```python
from build123d import *

# Parameters (mm, degrees)
SKETCH1_W           = 40
SKETCH1_H           = 25
BOSS_EXTRUDE1_DEPTH = 2
CUT_EXTRUDE1_REACH  = 25.67
SKETCH2_R           = 1.55


with BuildPart() as part:
    # Sketch1 → Boss-Extrude1 (new body)
    with BuildSketch(Plane.XY):
        Rectangle(SKETCH1_W, SKETCH1_H)
    extrude(amount=BOSS_EXTRUDE1_DEPTH)

    # Sketch2 → Cut-Extrude1 (cut, up to next)
    with BuildSketch(Plane.XY.offset(2), mode=Mode.PRIVATE) as cut_extrude1_sk1:
        with Locations((-15, 7.5)):
            Circle(SKETCH2_R)
    cut_extrude1_tool1 = extrude(cut_extrude1_sk1.sketch, amount=-CUT_EXTRUDE1_REACH, mode=Mode.PRIVATE) & part.part
    # Sketch2 → Cut-Extrude1 (cut, up to next)
    with BuildSketch(Plane.XY.offset(2), mode=Mode.PRIVATE) as cut_extrude1_sk2:
        with Locations((-15, 0)):
            Circle(SKETCH2_R)
    cut_extrude1_tool2 = extrude(cut_extrude1_sk2.sketch, amount=-CUT_EXTRUDE1_REACH, mode=Mode.PRIVATE) & part.part
    # Sketch2 → Cut-Extrude1 (cut, up to next)
    with BuildSketch(Plane.XY.offset(2), mode=Mode.PRIVATE) as cut_extrude1_sk3:
        with Locations((-15, -7.5)):
            Circle(SKETCH2_R)
    cut_extrude1_tool3 = extrude(cut_extrude1_sk3.sketch, amount=-CUT_EXTRUDE1_REACH, mode=Mode.PRIVATE) & part.part
    # Sketch2 → Cut-Extrude1 (cut, up to next)
    with BuildSketch(Plane.XY.offset(2), mode=Mode.PRIVATE) as cut_extrude1_sk4:
        with Locations((15, -7.5)):
            Circle(SKETCH2_R)
    cut_extrude1_tool4 = extrude(cut_extrude1_sk4.sketch, amount=-CUT_EXTRUDE1_REACH, mode=Mode.PRIVATE) & part.part
    # Sketch2 → Cut-Extrude1 (cut, up to next)
    with BuildSketch(Plane.XY.offset(2), mode=Mode.PRIVATE) as cut_extrude1_sk5:
        with Locations((15, 0)):
            Circle(SKETCH2_R)
    cut_extrude1_tool5 = extrude(cut_extrude1_sk5.sketch, amount=-CUT_EXTRUDE1_REACH, mode=Mode.PRIVATE) & part.part
    # Sketch2 → Cut-Extrude1 (cut, up to next)
    with BuildSketch(Plane.XY.offset(2), mode=Mode.PRIVATE) as cut_extrude1_sk6:
        with Locations((15, 7.5)):
            Circle(SKETCH2_R)
    cut_extrude1_tool6 = extrude(cut_extrude1_sk6.sketch, amount=-CUT_EXTRUDE1_REACH, mode=Mode.PRIVATE) & part.part
    add(cut_extrude1_tool1.solids().sort_by_distance((-15, 7.5, 2))[0], mode=Mode.SUBTRACT)
    add(cut_extrude1_tool2.solids().sort_by_distance((-15, 0, 2))[0], mode=Mode.SUBTRACT)
    add(cut_extrude1_tool3.solids().sort_by_distance((-15, -7.5, 2))[0], mode=Mode.SUBTRACT)
    add(cut_extrude1_tool4.solids().sort_by_distance((15, -7.5, 2))[0], mode=Mode.SUBTRACT)
    add(cut_extrude1_tool5.solids().sort_by_distance((15, 0, 2))[0], mode=Mode.SUBTRACT)
    add(cut_extrude1_tool6.solids().sort_by_distance((15, 7.5, 2))[0], mode=Mode.SUBTRACT)


solid = part.part
```
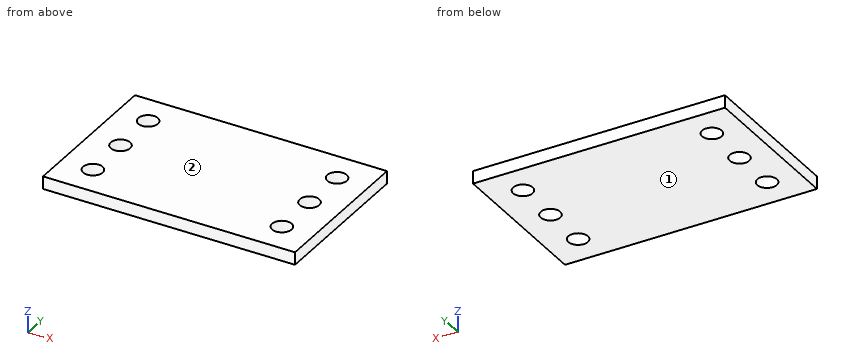
Can you work these out from the model? Positions are in its coordinate system, mm. Face numbers are marked on the shaded views. Coordinates: 2 decimals unless noted, no trailing zeros. Order: outer loops, then holes, each group sorted by start corner. A loop starts at its lowest first (then second) coordinate and runs counter-clockwise, first axis right, second up.
1. Thinking about a two-plate mould opening in Z: for the marked faces 1 and 2, which applies, +Z half, -Z half, draft (parallel to the pull), parting line (faces both ways), or undercut?
2. If we section it at C-C (z = 0.9): Please give me the cut outline in (x, y).
3. If we section it at B-B (y = 7.5): Please give me the cut outline in (x, z), then the cut area to 3 significant figures.
4. I'm going to push a flat-ended pin straight in: pin 1 (3 mm diameter, centred on x = -15, y = -7.5, fed in from +Z). Where does the tip first touch, or does it pass through?
5. If we section it at A-A (x = -15): Please give me the cut outline in (y, z).
6. I need wall thicknesses on line 1 (Y direction, x = -15, z = 1.55); line 2 (X direction, y = -0.5, z = 0.8); line 3 (Y direction, x = -14, z = 0.8). Which ranges of each line are inside material? Lowest first, please.
Entries:
1. face 1: -Z half
1. face 2: +Z half
2. outline: (-20, -12.5) - (20, -12.5) - (20, 12.5) - (-20, 12.5) - close; hole circle Ø3.1 at (-15, -7.5); hole circle Ø3.1 at (-15, 0); hole circle Ø3.1 at (-15, 7.5); hole circle Ø3.1 at (15, -7.5); hole circle Ø3.1 at (15, 0); hole circle Ø3.1 at (15, 7.5)
3. outline: (-20, 0) - (-16.55, 0) - (-16.55, 2) - (-20, 2) - close; (-13.45, 0) - (13.45, 0) - (13.45, 2) - (-13.45, 2) - close; (16.55, 0) - (20, 0) - (20, 2) - (16.55, 2) - close
3. area: 67.6 mm2
4. pin 1: passes through
5. outline: (-12.5, 0) - (-9.05, 0) - (-9.05, 2) - (-12.5, 2) - close; (-5.95, 0) - (-1.55, 0) - (-1.55, 2) - (-5.95, 2) - close; (1.55, 0) - (5.95, 0) - (5.95, 2) - (1.55, 2) - close; (9.05, 0) - (12.5, 0) - (12.5, 2) - (9.05, 2) - close
6. line 1: y = -12.5 to -9.05, -5.95 to -1.55, 1.55 to 5.95, 9.05 to 12.5
6. line 2: x = -20 to -16.47, -13.53 to 13.53, 16.47 to 20
6. line 3: y = -12.5 to -8.68, -6.32 to -1.18, 1.18 to 6.32, 8.68 to 12.5
